Geometry check sheet. Reference: drawing and pictorial views, mm from the part's lowest x, y, z. A direction names the side the tool comes from. Give positions to 0.01 mm unless a question says otherwise; leave off trailing zeros. Write each loop counter-clockwise with the first axis right and the second up, starting at its lowest first coordinate (ties: lowest second). Pieces come first, ordered by that corner, then holes. Notation, with made-up numbers: M 45,70.25 L 84,70.25 A6 ccw 84,75.25 Z; hole C 23,34.5 d9. An arc over 180 degrees is marked long. Write item = value, one per line. Start each with the question number.
1) Mould release check, pull along X, two halves, no side actions. Record for the marked faces 1, 2 and 3: released by +X, released by -X, zero draft, split by the parting line, or undercut.
2) Scan lines: line 1 along Z through (x, y) = (90, 13); line 2 along Y through (x, z) = (151, 106); line 3 along Z through (x, y) = (99, 44). Record each from-to range of solid material in increasing order. Write a range as [from, to].
3) Cross-section at C-C, the plane y = 16. Record the cut outline in (x, z), plus the area to 3 significant figures.
4) Access from +Z, -Z, +X, -X, +Y, -Y to the whole of each face (thin tool, end or side, straight path). Record for the marked faces 4 and 5.
5) Go/stop test with flat-tipped pins: pin 1 (12 mm diameter, centred on y = 35, z = 43.5, fed in from +X); pin 2 (12 mm diameter, centred on y = 36.5, z = 106, fed in from +X); pin 3 (4 mm diameter, centred on y = 16.5, z = 105, fed in from -X). Record where each tip stops, or that it passes through.
6) Cross-section at B-B, the plane z = 90. Record the cut outline in (x, y), plus the area to 3 significant figures.
7) Cross-section at D-D, the plane x = 59. Record the cut outline in (y, z), plus the area to 3 significant figures.
8) Cross-section at A-A, the plane x = 90. Record the cut outline in (y, z), plus the area to 3 significant figures.
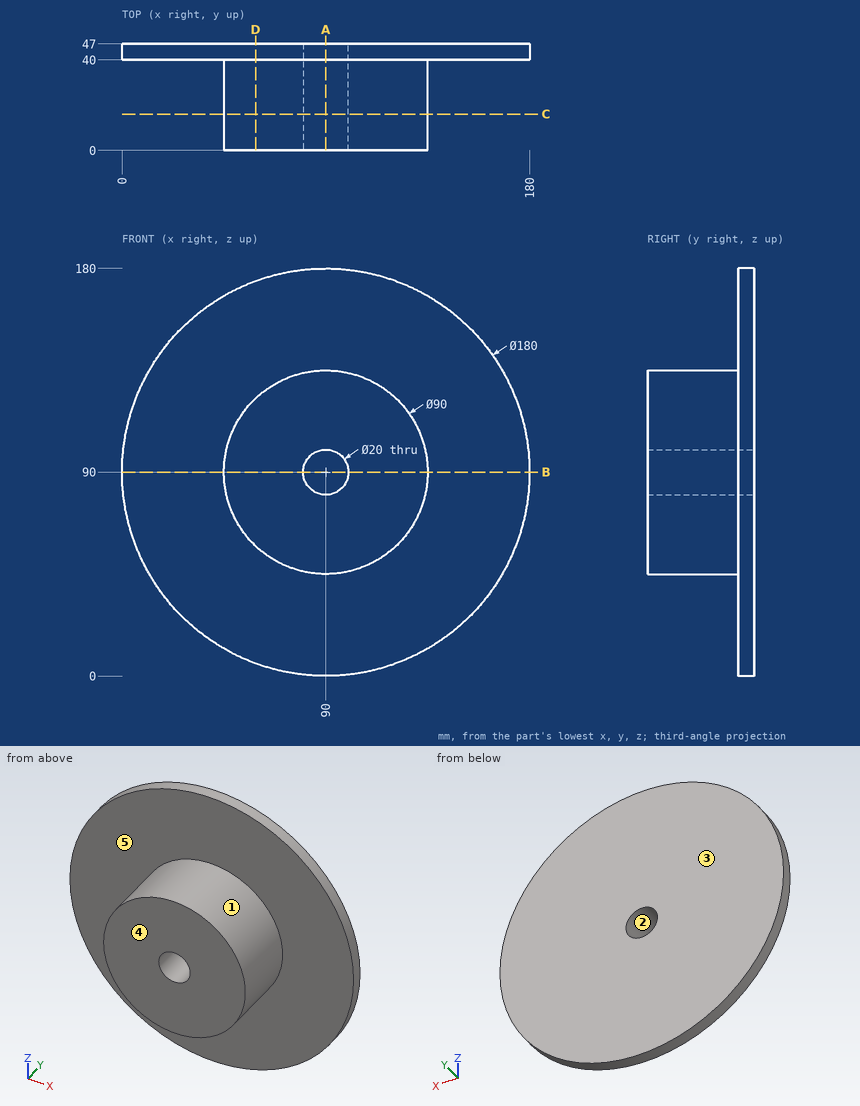
Reply:
q1.face_1 = split by the parting line
q1.face_2 = undercut
q1.face_3 = zero draft
q2.line_1 = [45, 80], [100, 135]
q2.line_2 = [40, 47]
q2.line_3 = [0.45, 85.64], [94.36, 179.55]
q3.outline = C 90,90 d90; hole C 90,90 d20
q3.area = 6,050 mm2
q4.face_4 = +Z, -Z, +X, -X, -Y
q4.face_5 = -Y
q5.pin_1 = 168.96
q5.pin_2 = 179.31
q5.pin_3 = 46.92
q6.outline = M 0,40 L 45,40 L 45,0 L 80,0 L 80,47 L 0,47 Z; M 100,0 L 135,0 L 135,40 L 180,40 L 180,47 L 100,47 Z
q6.area = 3,920 mm2
q7.outline = M 0,57.38 L 40,57.38 L 40,5.51 L 47,5.51 L 47,174.49 L 40,174.49 L 40,122.62 L 0,122.62 Z
q7.area = 3,790 mm2
q8.outline = M 0,45 L 40,45 L 40,0 L 47,0 L 47,80 L 0,80 Z; M 0,100 L 47,100 L 47,180 L 40,180 L 40,135 L 0,135 Z
q8.area = 3,920 mm2
